Check sheet for the modelled part. Datum: model origin and axes. Units: mm. Give positions to 0.01 mm unless a question says otherwise; leave off trailing zeros. Order: outer loops, then holes, each group sorted by start corner. A loop starts at its lowest first (then second) coordinate and runs counter-clockwise, first axis right, second up.
```python
from build123d import *

# Parameters (mm, degrees)
F0_W     = 50.8
F0_H     = 50.8
F0_R     = 2.38125
F0_R_2   = 15.5321
F1_DEPTH = 18.0086


with BuildPart() as f1:
    # F0 (on Top) → F1 (new body)
    with BuildSketch(Plane.XY):
        Rectangle(F0_W, F0_H)
        with Locations((-16.954631, -16.954631)):
            Circle(F0_R, mode=Mode.SUBTRACT)
        Circle(F0_R_2, mode=Mode.SUBTRACT)
        with Locations((16.954631, -16.954631)):
            Circle(F0_R, mode=Mode.SUBTRACT)
        with Locations((-16.954631, 16.954631)):
            Circle(F0_R, mode=Mode.SUBTRACT)
        with Locations((16.954631, 16.954631)):
            Circle(F0_R, mode=Mode.SUBTRACT)
    extrude(amount=F1_DEPTH)


solid = f1.part
```
(1) Cross-section at A-A on x = 0. Enter the section's corners in (y, z).
Response values:
outline: (-25.4, 0) - (-15.53, 0) - (-15.53, 18.01) - (-25.4, 18.01) - close; (15.53, 0) - (25.4, 0) - (25.4, 18.01) - (15.53, 18.01) - close
(2) Cross-section at B-B on y = -5.5. Enter the section's corners in (x, z), then the cut area to 3 significant figures.
Response values:
outline: (-25.4, 0) - (-14.53, 0) - (-14.53, 18.01) - (-25.4, 18.01) - close; (14.53, 0) - (25.4, 0) - (25.4, 18.01) - (14.53, 18.01) - close
area: 392 mm2
(3) Release check for a two-part mould opening along Y. For faces 1 (the face through (25.4, 0, 9)), 2 (the face through (19.226, 17.67, 8.878)), 3 (the face through (7.17, -13.78, 8.88)), 4 (the face through (0, 25.4, 9)) record: released by +Y, released by -Y, zero draft, split by the parting line, or undercut.
Response values:
face 1: zero draft
face 2: undercut
face 3: undercut
face 4: released by +Y
(4) Cross-section at D-D on z = 3.5. Enter the section's corners in (x, y), then the cut area to 3 significant figures.
Response values:
outline: (-25.4, -25.4) - (25.4, -25.4) - (25.4, 25.4) - (-25.4, 25.4) - close; hole circle Ø4.76 at (-16.95, -16.95); hole circle Ø4.76 at (-16.95, 16.95); hole circle Ø31.06 at (0, 0); hole circle Ø4.76 at (16.95, -16.95); hole circle Ø4.76 at (16.95, 16.95)
area: 1,750 mm2
(5) Gauge pin test, flat ends, axial feed: pin 1 Ø3 at (x, y) = (-16.95, 16.95) entering from -Z; pin 2 Ø7.5 at (x, y) = (16.95, 16.95) entering from -Z. Record the tip position at first contact, or that the pin passes through.
Response values:
pin 1: passes through
pin 2: stops at z = 0
(6) Cross-section at C-C on y = 18.5. Enter the section's corners in (x, z), then the cut area to 3 significant figures.
Response values:
outline: (-25.4, 0) - (-18.77, 0) - (-18.77, 18.01) - (-25.4, 18.01) - close; (-15.14, 0) - (15.14, 0) - (15.14, 18.01) - (-15.14, 18.01) - close; (18.77, 0) - (25.4, 0) - (25.4, 18.01) - (18.77, 18.01) - close
area: 784 mm2
(7) Material ranges on L1, parallel to Y at x = -18.5, z = 3.5; L2, parallel to X at y = 19, z = 8.75, recorded low to high.
Response values:
L1: y = -25.4 to -18.77, -15.14 to 15.14, 18.77 to 25.4
L2: x = -25.4 to -18.17, -15.74 to 15.74, 18.17 to 25.4
